Input: part model. Units: mm. Frame: model coordinates. Face numbers are marked on the shaded views. Give positions to 0.01 mm unless a question says otherwise; leave off trailing zeros. Loops run counter-clockwise (first coordinate to the right, second up) from the corner with the lowest first, then second, coordinate; pieces in that order, holes last. Notation, with made-up numbers: M 54.5,60 L 95.5,60 A9 ccw 95.5,66 Z; hole C 69.5,-18 d11. An arc over 180 degrees is marked long. Use a Markdown table: item, result. Add a question column.
from build123d import *

# Parameters (mm, degrees)
SKETCH1_R                           = 22.86
BOSS_EXTRUDE1_DEPTH                 = 6.35
BOSS_EXTRUDE2_DEPTH                 = 8.89
SKETCH3_R                           = 10.795
BOSS_EXTRUDE3_DEPTH                 = 304.8
CHAMFER1_SIZE                       = 3.81
F_5_32_0_15625_DIAMETER_HOLE1_D     = 3.96875
F_5_32_0_15625_DIAMETER_HOLE1_DEPTH = 6.351
CIRPATTERN1_COUNT                   = 4
SKETCH7_W                           = 70.612
SKETCH7_H                           = 52.07
BOSS_EXTRUDE4_DEPTH                 = 60.96
SKETCH8_R                           = 7.112
CUT_EXTRUDE1_DEPTH                  = 71.612


with BuildPart() as part:
    # Sketch1 → Boss-Extrude1 (new body)
    with BuildSketch(Plane(origin=(0, 0, 0), x_dir=(1, 0, 0), z_dir=(0, 1, 0))):
        Circle(SKETCH1_R)
    extrude(amount=BOSS_EXTRUDE1_DEPTH)

    # Sketch2 → Boss-Extrude2 (add)
    with BuildSketch(Plane(origin=(0, 6.35, 0), x_dir=(1, 0, 0), z_dir=(0, 1, 0))):
        with BuildLine():
            Line((1.9685, -4.266803107), (1.9685, 4.266803107))
            ThreePointArc((1.9685, 4.266803107), (0, 4.699), (-1.9685, 4.266803107))
            Line((-1.9685, 4.266803107), (-1.9685, -4.266803107))
            ThreePointArc((-1.9685, -4.266803107), (0, -4.699), (1.9685, -4.266803107))
        make_face()
    extrude(amount=BOSS_EXTRUDE2_DEPTH)

    # Sketch3 → Boss-Extrude3 (add)
    with BuildSketch(Plane.XZ):
        Circle(SKETCH3_R)
    extrude(amount=BOSS_EXTRUDE3_DEPTH)

    # Chamfer1
    chamfer1_edges = [part.edges().sort_by_distance(p)[0] for p in [
        (-10.795, 0, 0),
    ]]
    chamfer(chamfer1_edges, length=CHAMFER1_SIZE)

    # 5/32 (0.15625) Diameter Hole1
    with Locations(Plane(origin=(0, 6.35, 0), x_dir=(1, 0, 0), z_dir=(0, 1, 0))):
        with Locations((0, 18)):
            f_5_32_0_15625_diameter_hole1 = Hole(F_5_32_0_15625_DIAMETER_HOLE1_D / 2, depth=F_5_32_0_15625_DIAMETER_HOLE1_DEPTH)

    # CirPattern1: 5/32 (0.15625) Diameter Hole1 ×4 about axis
    cirpattern1_axis = Axis((0, 0, 0), (0, 1, 0))
    for i in range(1, CIRPATTERN1_COUNT):
        add(f_5_32_0_15625_diameter_hole1.rotate(cirpattern1_axis, i * 360 / CIRPATTERN1_COUNT), mode=Mode.SUBTRACT)

    # Sketch7 → Boss-Extrude4 (add)
    with BuildSketch(Plane.XZ.offset(304.8)):
        Rectangle(SKETCH7_W, SKETCH7_H)
    extrude(amount=BOSS_EXTRUDE4_DEPTH)

    # Sketch8 → Cut-Extrude1 (cut, through all)
    with BuildSketch(Plane(origin=(35.306, 0, 0), x_dir=(0, 0, -1), z_dir=(1, 0, 0))):
        with Locations((0, -335.28)):
            Circle(SKETCH8_R)
    extrude(amount=-CUT_EXTRUDE1_DEPTH, mode=Mode.SUBTRACT)


solid = part.part
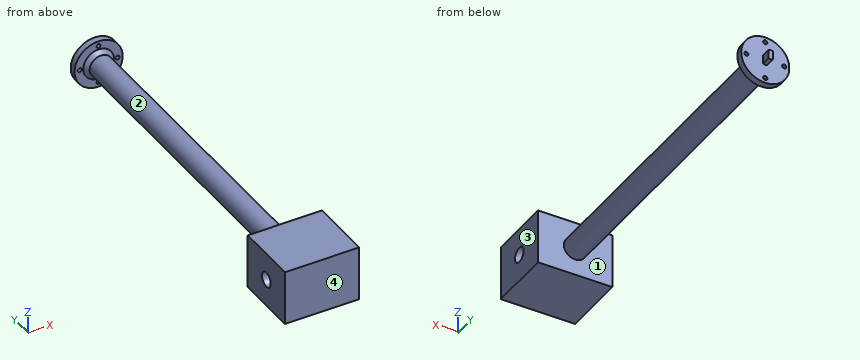
1) Section query C-C, the plane y = -9. Return the cut outline in (x, z) (3 decimals), and give its area (3 significant figures).
2) Section query B-B, the plane x = 30. Return the cut outline in (y, z) (3 decimals), and give its area (3 significant figures).
3) Pull-direction query (Y, two-part tool) for the marked faces 1, 2, 3 and 4; classes: pulls with the +Y half, pulls with the -Y half, needs draft (parallel to the pull), parting line crosses it, or undercut.
4) Ray query, line 1 (Y direction, x = -16, z = 1); line 2 (X direction, y = 3, z = 0). Return the intervals inside material, ascending. Write a range as [from, to].
5) Section query A-A, the plane y = -335.28. Return the cut outline in (x, z) (3 decimals).
6) Contact query for flat-ended pins moving along their axis: P1, Ø8, axis at x = 9.5, y = -199, coming from the -Z side; P2, Ø15.5, axis at x = -5, z = 2.5, coming from the +Y side; P3, Ø8, axis at x = 5, y = -292, coming from the +Z side; P4, Ø10, axis at y = -226, z = -7.5, coming from the +X side. Output: stop coordinate, or through.
Entries:
| question | item | result |
|---|---|---|
| 1 | outline | C 0,0 d21.59 |
| 1 | area | 366 mm² |
| 2 | outline | M -365.76,-26.035 L -304.8,-26.035 L -304.8,26.035 L -365.76,26.035 Z; hole C -335.28,0 d14.224 |
| 2 | area | 3,020 mm² |
| 3 | face 1 | undercut |
| 3 | face 2 | undercut |
| 3 | face 3 | needs draft |
| 3 | face 4 | pulls with the -Y half |
| 4 | line 1 | y = [-365.76, -342.32], [-328.24, -304.8], [0, 6.35] |
| 4 | line 2 | x = [-22.86, -19.98], [-16.02, 16.02], [19.98, 22.86] |
| 5 | outline | M -35.306,-26.035 L 35.306,-26.035 L 35.306,-7.112 L -35.306,-7.112 Z; M -35.306,7.112 L 35.306,7.112 L 35.306,26.035 L -35.306,26.035 Z |
| 6 | P1 | stops at z = -9.29 |
| 6 | P2 | stops at y = 15.24 |
| 6 | P3 | stops at z = 10.75 |
| 6 | P4 | stops at x = 10.5 |
